from build123d import *

# Parameters (mm, degrees)
SKETCH_1_W          = 100
SKETCH_1_H          = 80
EXTRUDE_1_DEPTH     = 100
FILLET_1_R          = 20
FILLET_2_R          = 10
CUT_EXTRUDE_1_DEPTH = 5


with BuildPart() as part:
    # Эскиз1 → Бобышка-Вытянуть1 (new body)
    with BuildSketch(Plane.XY):
        with Locations((50, 40)):
            Rectangle(SKETCH_1_W, SKETCH_1_H)
    extrude(amount=EXTRUDE_1_DEPTH)

    # Скругление1
    fillet_1_edges = [part.edges().sort_by_distance(p)[0] for p in [
        (100, 0, 50),
        (0, 0, 50),
        (0, 80, 50),
        (100, 80, 50),
    ]]
    fillet(fillet_1_edges, radius=FILLET_1_R)

    # Скругление2
    fillet_2_edges = [part.edges().sort_by_distance(p)[0] for p in [
        (50, 80, 0),
        (50, 80, 100),
        (100, 40, 0),
        (50, 0, 0),
        (0, 40, 0),
        (5.857864376, 5.857864376, 0),
        (5.857864376, 74.142135624, 0),
        (94.142135624, 5.857864376, 0),
        (94.142135624, 74.142135624, 0),
        (100, 40, 100),
        (0, 40, 100),
        (50, 0, 100),
        (5.857864376, 5.857864376, 100),
        (5.857864376, 74.142135624, 100),
        (94.142135624, 5.857864376, 100),
        (94.142135624, 74.142135624, 100),
    ]]
    fillet(fillet_2_edges, radius=FILLET_2_R)

    # Эскиз2 → Вырез-Вытянуть1 (cut)
    with BuildSketch(Plane.XZ):
        with BuildLine():
            Line((20, 10), (80, 10))
            add(Edge.make_bspline(
                [(80, 10), (80, 80), (50, 80), (20, 80), (20, 10)],
                knots=[4.71238898, 4.71238898, 4.71238898, 6.283185307, 6.283185307, 7.853981634, 7.853981634, 7.853981634], degree=2, weights=[1, 0.707106781, 1, 0.707106781, 1]))
        make_face()
    extrude(amount=-CUT_EXTRUDE_1_DEPTH, mode=Mode.SUBTRACT)


solid = part.part
Read the model definition and answer for the solid it produces. Units are mm, in the model's axes. A direction names the side the tool comes from. Round coordinates to 2 decimals unless told otherwise and drop trailing zeros. Loops run counter-clockwise (first coordinate to the right, second up) from the corner with the lowest first, then second, coordinate; pieces in that order, holes last.
Q1. Determine the mould class of faces 3 (the face through (50, 2, 10)), 4 (the face through (50, 80, 49)), 5 (the face through (5.703, 6.014, 50.56)) for opening direction X: released by +X, released by -X, zero draft, split by the parting line, or undercut.
Q2. Consider probe 1 along X at (y, z) = (61, 35); probe 2 along Y at (x, z) = (48.5, 31); probe 3 along X at (y, z) = (73, 42). Determine where each line is inside the solid, lowest interval first.
Q3. Section A-A on z = 84 is taken. Write down the section's boundary in (x, y), and give its area (3 significant figures).
Q4. Each of these flat-tipped pins is pushed along its axis until it touches: pin 1 (1.5 mm diameter, centred on x = 44.5, y = 2.5, fed in from +Z); pin 2 (1.5 mm diameter, centred on y = 69, z = 45.5, fed in from -X). Where does it stop, or does it pass through?
Q5. Which of the six approach directions +Z, -Z, +X, -X, +Y, -Y give full straight-line access (tool end or side, diameter ignored) to faces 1 (the face through (49.58, 3.01, 97.15)), 2 (the face through (50, 5, 38))?
Output:
1. face 3: undercut
1. face 4: zero draft
1. face 5: released by -X
2. probe 1: x = 0.03 to 99.97
2. probe 2: y = 5 to 80
2. probe 3: x = 4.8 to 95.2
3. outline: (0, 20) arc R20 ccw to (20, 0) - (80, 0) arc R20 ccw to (100, 20) - (100, 60) arc R20 ccw to (80, 80) - (20, 80) arc R20 ccw to (0, 60) - close
3. area: 7,660 mm2
4. pin 1: stops at z = 97.38
4. pin 2: stops at x = 1.78
5. face 1: +Z, +X, -X, -Y
5. face 2: -Y
